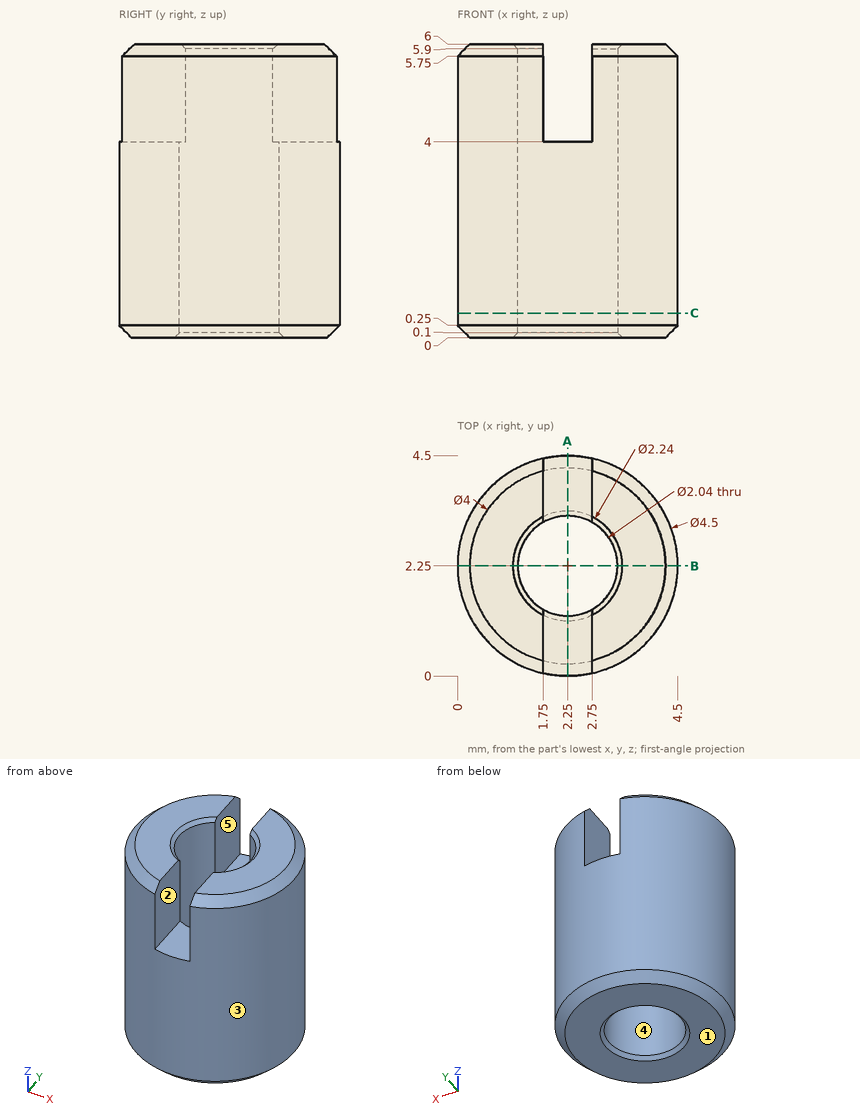
Here's the drawing with two shaded views (mm, measured from the low corner). I have some questions. A direction names the side the tool comes from. Coordinates: 2 decimals unless noted, no trailing zeros. Order: outer loops, then holes, each group sorted by start corner. A loop starts at its lowest first (then second) coordinate and runs counter-clockwise, first axis right, second up.
Q1. Which directions (+Z, -Z, +X, -X, +Y, -Y) give clear straight access to the entire face, cutting with the end or side of a thin tool? Please do the marked faces 4 and 5.
Q2. Suppose I cut it at A-A on x = 2.25. Please give me the cut outline in (y, z).
Q3. Suppose I cut it at B-B on y = 2.25. Please give me the cut outline in (x, z).
Q4. Thinking about a two-plate mould opening in X: for the marked faces 1, 2 and 3, which applies, released by +X, released by -X, zero draft, split by the parting line, or undercut?
Q5. Please list where these lines run through material, in increasing order: L1, parallel to Y at x = 2.25, z = 3.35; L2, parallel to X at y = 2.75, z = 3; L3, parallel to Z at x = 2, y = 3.7.
Q6. Will these pins go through, and if not, where does the flat tip stop? pin 1 (1 mm diameter, centred on y = 4, z = 4.5, fed in from +X); pin 2 (1.4 mm diameter, centred on y = 4, z = 5, fed in from -X); pin 3 (1.8 mm diameter, centred on x = 2.25, y = 2.25, fed in from -Z); pin 4 (1.5 mm diameter, centred on x = 3.5, z = 3, fed in from +Y).
Q7. Suppose I cut it at C-C on z = 0.5. Please give me the cut outline in (x, y), and give its area (3 significant figures).
Answer:
1. face 4: +Z, -Z
1. face 5: +Z, +Y, -Y
2. outline: (0, 0.25) - (0.25, 0) - (1.13, 0) - (1.23, 0.1) - (1.23, 4) - (0, 4) - close; (3.27, 0.1) - (3.37, 0) - (4.25, 0) - (4.5, 0.25) - (4.5, 4) - (3.27, 4) - close
3. outline: (0, 0.25) - (0.25, 0) - (1.13, 0) - (1.23, 0.1) - (1.23, 5.9) - (1.13, 6) - (0.25, 6) - (0, 5.75) - close; (3.27, 0.1) - (3.37, 0) - (4.25, 0) - (4.5, 0.25) - (4.5, 5.75) - (4.25, 6) - (3.37, 6) - (3.27, 5.9) - close
4. face 1: zero draft
4. face 2: undercut
4. face 3: split by the parting line
5. L1: y = 0 to 1.23, 3.27 to 4.5
5. L2: x = 0.06 to 1.36, 3.14 to 4.44
5. L3: z = 0 to 4
6. pin 1: stops at x = 4.12
6. pin 2: stops at x = 0.26
6. pin 3: passes through
6. pin 4: stops at y = 4.44
7. outline: circle Ø4.5 at (2.25, 2.25); hole circle Ø2.04 at (2.25, 2.25)
7. area: 12.6 mm2
